Autodesk Inventor part; units mm, degrees
ref_plane "Start Plane" through (0, 0, 70.7107) normal (0, 0, 1) x (1, 0, 0)
ref_plane "End Plane" through (0, 0, 1829.2893) normal (0, 0, 1) x (1, 0, 0)
ref_plane "Work Plane4" through (0, 20, 1829.2893) normal (0, -0.3827, 0.9239) x (1, 0, 0)
ref_plane "Start Plane" through (0, 0, 70.7107) normal (0, 0, 1) x (1, 0, 0)
ref_plane "End Plane" through (0, 0, 1829.2893) normal (0, 0, 1) x (1, 0, 0)
sketch "Sketch" plane through (0, 0, 0) normal (0, 0, 1) x (1, 0, 0)
  line L0 (-10, -16) -> (-10, 16)
  line L1 (-6, 20) -> (6, 20)
  line L2 (10, 16) -> (10, -16)
  line L3 (6, -20) -> (-6, -20)
  arc A0 (-10, -16) -> (-6, -20) centre (-6, -16) ccw
  arc A1 (10, 16) -> (6, 20) centre (6, 16) ccw
  arc A2 (-6, 20) -> (-10, 16) centre (-6, 16) ccw
  arc A3 (6, -20) -> (10, -16) centre (6, -16) ccw
  arc A4 (-6, 18) -> (-8, 16) centre (-6, 16) ccw
  line L4 (-6, 18) -> (6, 18)
  arc A5 (8, 16) -> (6, 18) centre (6, 16) ccw
  line L5 (8, 16) -> (8, -16)
  arc A6 (6, -18) -> (8, -16) centre (6, -16) ccw
  line L6 (6, -18) -> (-6, -18)
  arc A7 (-8, -16) -> (-6, -18) centre (-6, -16) ccw
  line L7 (-8, -16) -> (-8, 16)
  line L8 (0, 29.1598) -> (0, -29.1598) construction
  line L9 (-15.1598, 0) -> (15.1598, 0) construction
  dimension "d7" = 4
  dimension "d9" = 20
  dimension "d11" = 40
  dimension "d12" = 2
  dimension "d15" = 10
  dimension "d16" = 20
extrude "Body" add sketch "Sketch" along normal up to surface (1758.5786 mm away) from surface at 70.7107
sketch "Sketch3" plane through (0, 0, 0) normal (0, 0, 1) x (1, 0, 0)
  line L0 (0, 0) -> (10, 0)
ref_plane "Work Plane3" through (0, 0, 0) normal (0, -1, 0) x (1, 0, 0)
ref_plane "Work Plane4" through (0, 20, 1829.2893) normal (0, -0.3827, 0.9239) x (1, 0, 0)
split "Split1" plane through (0, 20, 1829.2893) removes the side toward (0, -0.3827, 0.9239)
ref_plane "Work Plane5" through (0, 20, 70.7107) normal (0, -0.3827, -0.9239) x (1, 0, 0)
split "Split2" plane through (0, 20, 70.7107) removes the side toward (0, -0.3827, -0.9239)
sketch "Sketch5" plane through (-10, 16, 72.3675) normal (-1, 0, 0) x (0, 0, 1)
  line L0 (0, 0) -> (13.2548, -32) construction
  line L1 (13.2548, -32) -> (1742.0101, -32) construction
  line L2 (1742.0101, -32) -> (1755.2649, 0) construction
  line L3 (0, 0) -> (1755.2649, 0) construction
  line L4 (877.6325, -32) -> (877.6325, 0) construction
  line L5 (877.6325, -16) -> (1748.6375, -16) construction
  line L6 (877.6325, -16) -> (6.6274, -16) construction
  circle A0 centre (1227.6325, -16) radius 5.5
  circle A1 centre (927.6325, -16) radius 5.5
  circle A2 centre (1327.6325, -16) radius 5.5
  circle A3 centre (1627.6325, -16) radius 5.5
  point P0 (-72.3675, -16)
  dimension "d19" = 11
  dimension "d20" = 300
  dimension "d21" = 50
  dimension "d22" = 300
  dimension "d23" = 100
extrude "Extrusion2" cut sketch "Sketch5" against normal up to surface (2 mm away)
sketch "Sketch4" plane through (0, 0, 0) normal (0, -1, 0) x (1, 0, 0)
  line L0 (-2, 70.7107) -> (12, 70.7107)
  line L1 (-2, 1829.2893) -> (12, 1829.2893)
  dimension "d18" = 1758.5786
equation "\"d7\" = G_IR"
equation "\"d9\" = G_W"
equation "\"d11\" = G_H"
equation "\"d12\" = G_T"
equation "\"d15\" = 0.5 * d9"
equation "\"d16\" = 0.5 * d11"
equation "\"d3\" = G_L"
equation "\"d22\" = d20"
equation "\"G_W\" = 20"
equation "\"G_H\" = 40"
equation "\"G_T\" = 2"
equation "\"G_IR\" = 4"
equation "\"G_L\" = d18"
equation "\"G_OFFSET_START\" = -70.71068"
equation "\"G_OFFSET_END\" = -70.71068"
equation "\"d13\" = -G_OFFSET_START"
equation "\"d14\" = G_OFFSET_END + B_L"
properties part number "ISO 4019 - 40x20x2 - 1758,58" material "Steel, Mild"
Design review of the part built by this model. Coordinates are the model's own, in mm. Round coordinates to 2 decimals unless told otherwise and drop trailing zeros. Write each loop counter-clockwise with the first axis right and the second up, starting at its lowest first coordinate (ties: lowest second). Pieces come first, ordered by that corner, then holes. Notation, with made-up numbers: M 32,19.25 L 47,19.25 A19 cw 47,55.25 Z; hole C 72.5,61.5 d1. An arc over 180 degrees is marked long. One line per item, written item: value. Start each with the question number.
1. Draft analysis for pull direction X (two halves, no side actions). For faces 1 (the face through (10, 0, 938)), 2 (the face through (-8, 0, 938)), 3 (the face through (-10, 0, 938)), state which applies: pulls with the +X half, pulls with the -X half, needs draft (parallel to the pull), parting line crosses it, or undercut.
2. Take a section at A-A on z = 247.5. State the section outline as (x, y) points.
3. Clearance check with flat-ended pins moving along their axes: P1, Ø14.5, axis at y = 0, z = 1000, coming from the -X side; P2, Ø9, axis at y = 0, z = 1300, coming from the -X side; P3, Ø12, axis at x = -2.5, y = -3, coming from the +Z side. State where each tip first meets the part, or that it passes through.
4. Take a section at B-B on x = 2. State the section outline as (y, z) points, then the cut area to 3 significant figures.
5. To check wall thickness, follow probe 1 along X at (y, z) = (10.5, 1116.5); probe 2 along Y at (x, z) = (-6, 1243.5); probe 3 along X at (y, z) = (-16.5, 870). State the ranges of each line that lie inside material, in increasing order. Write a range as from..to.
Computed:
1. face 1: pulls with the +X half
1. face 2: undercut
1. face 3: pulls with the -X half
2. outline: M -10,-16 A4 ccw -6,-20 L 6,-20 A4 ccw 10,-16 L 10,16 A4 ccw 6,20 L -6,20 A4 ccw -10,16 Z; hole M -8,-16 A2 ccw -6,-18 L 6,-18 A2 ccw 8,-16 L 8,16 A2 ccw 6,18 L -6,18 A2 ccw -8,16 Z
3. P1: stops at x = -10
3. P2: stops at x = 8
3. P3: stops at z = 1820.76
4. outline: M -20,87.28 L -18,86.45 L -18,1813.55 L -20,1812.72 Z; M 18,71.54 L 20,70.71 L 20,1829.29 L 18,1828.46 Z
4. area: 6,970 mm²
5. probe 1: x = -10..-8, 8..10
5. probe 2: y = -20..-18, 18..20
5. probe 3: x = -9.97..-7.94, 7.94..9.97
